The listing builds one solid part. Answer for the finished solid, in the listing's coordinates (mm). Face numbers are marked on the shaded views. A direction names the side the tool comes from. Coordinates: 2 decimals unless noted, no trailing zeros. Write each loop counter-clockwise with the first axis right and the second up, starting at its lowest first coordinate (ties: lowest second). Pieces come first, ordered by that corner, then holes.
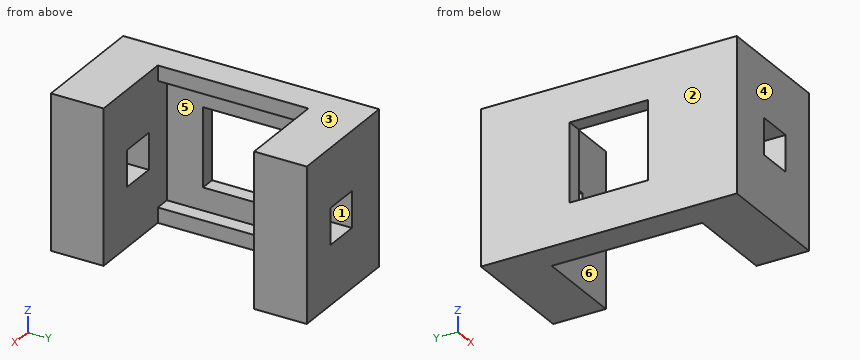
from build123d import *

# Parameters (mm, degrees)
SKETCH049_W      = 1
SKETCH049_H      = 1
EXTRUDE052_DEPTH = 8.5
SKETCH048_W      = 2.4
SKETCH048_H      = 2.4
EXTRUDE051_DEPTH = 8.5
SKETCH046_W      = 5.2
SKETCH046_H      = 5.2
EXTRUDE049_DEPTH = 1
SKETCH047_W      = 10
SKETCH047_H      = 10.2
EXTRUDE050_DEPTH = 8
SKETCH045_W      = 8
SKETCH045_H      = 10.2
EXTRUDE048_DEPTH = 8.5


with BuildPart() as extrude052:
    # Sketch049 → Extrude052 (new body, symmetric)
    with BuildSketch(Plane.XZ):
        with Locations((1.5, -4.6)):
            Rectangle(SKETCH049_W, SKETCH049_H)
        with Locations((1.5, 4.6)):
            Rectangle(SKETCH049_W, SKETCH049_H)
    extrude(amount=EXTRUDE052_DEPTH, both=True)


with BuildPart() as obj1:
    # Sketch048 → Extrude051 (new body, symmetric)
    with BuildSketch(Plane.XZ):
        with Locations((4.2, 0)):
            Rectangle(SKETCH048_W, SKETCH048_H)
    extrude(amount=EXTRUDE051_DEPTH, both=True)


with BuildPart() as obj2:
    # Sketch046 → Extrude049 (new body)
    with BuildSketch(Plane.YZ):
        Rectangle(SKETCH046_W, SKETCH046_H)
    extrude(amount=EXTRUDE049_DEPTH)


with BuildPart() as obj3:
    # Sketch047 → Extrude050 (new body)
    with BuildSketch(Plane.YZ):
        Rectangle(SKETCH047_W, SKETCH047_H)
    extrude(amount=EXTRUDE050_DEPTH)


with BuildPart() as obj3_1:
    # Extrude050 placement: moved
    add(obj3.part.moved(Location((1, 0, 0))))


with BuildPart() as obj4:
    # Sketch045 → Extrude048 (new body, symmetric)
    with BuildSketch(Plane.XZ):
        with Locations((4, 0)):
            Rectangle(SKETCH045_W, SKETCH045_H)
    extrude(amount=EXTRUDE048_DEPTH, both=True)

    # Cut030: cut obj3
    add(obj3_1.part, mode=Mode.SUBTRACT)

    # Cut031: cut obj2
    add(obj2.part, mode=Mode.SUBTRACT)

    # Cut032: cut obj1
    add(obj1.part, mode=Mode.SUBTRACT)

    # Fusion001: union Extrude052
    add(extrude052.part)


solid = obj4.part
1. Flat-ended cylindrical pins translate along their axes: P1, Ø1, axis at x = 3.5, y = 2.5, coming from the -Z side; P2, Ø4, axis at y = 0.5, z = 1, coming from the +X side. Find the tip coordinate at first contact, or state that the pin passes through.
Results found:
P1: passes through
P2: stops at x = 1
2. A tool of negligible diameter and unlimited length cuts with its end or side. For the marked faces 1 and 2, from which of +Z, -Z, +X, -X, +Y, -Y can it reach the whole face along a straight path? Write none if from no direction.
Results found:
face 1: +Y, -Y
face 2: +Z, -Z, -X, +Y, -Y
3. Section C-C on z = -2 is taken. Give the vertices of the cut face in (x, y).
Results found:
outline: (0, -8.5) - (8, -8.5) - (8, -5) - (1, -5) - (1, -2.6) - (0, -2.6) - close; (0, 2.6) - (1, 2.6) - (1, 5) - (8, 5) - (8, 8.5) - (0, 8.5) - close
4. Section B-B on y = -1 is taken. Give the vertices of the cut face in (x, z), then the cut area to 3 significant figures.
Results found:
outline: (0, -5.1) - (2, -5.1) - (2, -4.1) - (1, -4.1) - (1, -2.6) - (0, -2.6) - close; (0, 2.6) - (1, 2.6) - (1, 4.1) - (2, 4.1) - (2, 5.1) - (0, 5.1) - close
area: 7.00 mm2
5. Section A-A on x = 5 is taken. Give the vertices of the cut face in (y, z).
Results found:
outline: (-8.5, -5.1) - (-5, -5.1) - (-5, -1.2) - (-8.5, -1.2) - close; (-8.5, 1.2) - (-5, 1.2) - (-5, 5.1) - (-8.5, 5.1) - close; (5, -5.1) - (8.5, -5.1) - (8.5, -1.2) - (5, -1.2) - close; (5, 1.2) - (8.5, 1.2) - (8.5, 5.1) - (5, 5.1) - close
6. Find the intervals of material crossed by L1, parallel to X at y = -6.25, z = 0; L2, parallel to Y at x = 5.5, z = 3.75; L3, parallel to Y at x = 0.75, z = 1.75, in increasing order.
Results found:
L1: x = 0 to 3, 5.4 to 8
L2: y = -8.5 to -5, 5 to 8.5
L3: y = -8.5 to -2.6, 2.6 to 8.5
7. Section D-D on x = 6 is taken. Give the vertices of the cut face in (y, z).
Results found:
outline: (-8.5, -5.1) - (-5, -5.1) - (-5, 5.1) - (-8.5, 5.1) - close; (5, -5.1) - (8.5, -5.1) - (8.5, 5.1) - (5, 5.1) - close
8. For a pull along Y with two mould halves and no side action, classify the marked faces 3, 4, 5 and 6 as pulls with the +Y half, pulls with the -Y half, needs draft (parallel to the pull), parting line crosses it, or undercut.
Results found:
face 3: needs draft
face 4: pulls with the -Y half
face 5: undercut
face 6: undercut
